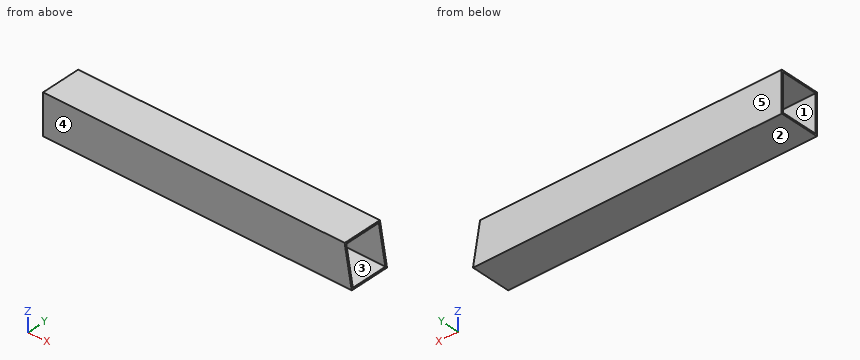
```python
from build123d import *

# Parameters (mm, degrees)
F0_W     = 65
F0_H     = 65
F1_DEPTH = 500
F2_W     = 60
F2_H     = 60
F3_DEPTH = 500
F5_DEPTH = 70


with BuildPart() as f1:
    # F0 (on Right) → F1 (new body)
    with BuildSketch(Plane.YZ):
        with Locations((25.129514, -17.626217)):
            Rectangle(F0_W, F0_H)
    extrude(amount=F1_DEPTH)

    # F2 (on face) → F3 (cut)
    with BuildSketch(Plane.YZ.offset(500)):
        with Locations((25.129514, -17.626217)):
            Rectangle(F2_W, F2_H)
    extrude(amount=-F3_DEPTH, mode=Mode.SUBTRACT)

    # F4 (on face) → F5 (cut)
    with BuildSketch(Plane.XZ.offset(7.370486)):
        Polygon((488.538746, 14.873783), (500, -50.126217), (500, 14.873783), align=None)
    extrude(amount=-F5_DEPTH, mode=Mode.SUBTRACT)


solid = f1.part
```
Can you work these out from the model? Positions are in its coordinate system, mm. Face numbers are marked on the shaded views. A direction names the side the tool comes from. Round coordinates to 2 decimals unless told otherwise and drop trailing zeros. Loops run counter-clockwise (first coordinate to the right, second up) from the corner with the lowest first, then second, coordinate; pieces in that order, holes last. Notation, with made-up numbers: M 58,49 L 74,49 A30 ccw 74,82 Z; hole C 38,41 d8. An arc over 180 degrees is marked long. Answer in a Markdown table with one row per item.
1. On a 3-axis mill with a long thin cutter (end or side, diameter ignored), from which of +Z, -Z, +X, -X, +Y, -Y can I reach the whole of each face in a straight line? I mean the marked faces 1 and 2. Say none if no direction works.
Established:
| item | result |
|---|---|
| face 1 | +X, -X |
| face 2 | -Z, +X, -X, +Y, -Y |
2. Please list where these lines run through material, in increasing order: line 1 (Z direction, x = 473, y = 53); line 2 (Y direction, x = 293, z = -8); line 3 (X direction, y = 30, z = 12.5). Write a range as from..to.
Established:
| item | result |
|---|---|
| line 1 | -50.13..-47.63, 12.37..14.87 |
| line 2 | -7.37..-4.87, 55.13..57.63 |
| line 3 | 0..488.96 |
3. Thinking about a two-plate mould opening in Y: for the marked faces 3, 4 and 5, which applies, pulls with the +Y half, pulls with the -Y half, needs draft (parallel to the pull), parting line crosses it, or undercut?
Established:
| item | result |
|---|---|
| face 3 | undercut |
| face 4 | pulls with the -Y half |
| face 5 | pulls with the +Y half |
4. I'm going to push a flat-ended pin straight in: pin 1 Ø12 at (y, z) = (6.5, -25.5) entering from +X. Where does the tip first touch, or does it pass through?
Established:
| item | result |
|---|---|
| pin 1 | through |
5. If we section it at A-A, the plane x = 84: Please give me the cut outline in (y, z).
Established:
| item | result |
|---|---|
| outline | M -7.37,-50.13 L 57.63,-50.13 L 57.63,14.87 L -7.37,14.87 Z; hole M -4.87,-47.63 L 55.13,-47.63 L 55.13,12.37 L -4.87,12.37 Z |
6. If we section it at B-B, the plane z = -37: Please give me the cut outline in (x, y), plus the area to 3 significant figures.
Established:
| item | result |
|---|---|
| outline | M 0,-7.37 L 497.69,-7.37 L 497.69,-4.87 L 0,-4.87 Z; M 0,55.13 L 497.69,55.13 L 497.69,57.63 L 0,57.63 Z |
| area | 2,490 mm² |
7. If we section it at C-C, the plane y = 35: Please give me the cut outline in (x, z).
Established:
| item | result |
|---|---|
| outline | M 0,-50.13 L 500,-50.13 L 499.56,-47.63 L 0,-47.63 Z; M 0,12.37 L 488.98,12.37 L 488.54,14.87 L 0,14.87 Z |
